Design review of the part shown in the three views and the two pictorial views. Dimensions are in mm from the part's minimum x, y and z. A direction names the side the tool comes from. Coordinates: 2 decimals unless noted, no trailing zeros. Loops run counter-clockwise (first coordinate to the right, second up) from the corner with the lowest first, then second, coordinate; pieces in that order, holes last.
Q1. Wall thickness on probe 1 along Y at (x, z) = (6, 42.5); probe 2 along X at (y, z) = (38, 43.5); probe 3 along Z at (x, y) = (6.5, 13): over which ranges is each line inside the solid? List them lowest first.
Q2. Add section D-D on y = 30. Give the boundary of the cut face in (x, z).
Q3. Add section C-C on z = 47. Give the boundary of the cut face in (x, y).
Q4. Add section A-A on y = 21.25. Give the boundary of the cut face in (x, z).
Q5. For P1, Ø10, axis at x = 22, y = 36.5, coming from the +Z side; P2, Ø3, axis at x = 5.755, y = 5.755, coming from the +Z side, all flat-tipped, find the tip position at first contact; note any pin that passes through.
Q6. Machinability: for the marked faces 1 and 2, which of the approach directions +Z, -Z, +X, -X, +Y, -Y give a long, thin tool a straight path to every point of the face, cutting with its end or side? Answer none if there is none.
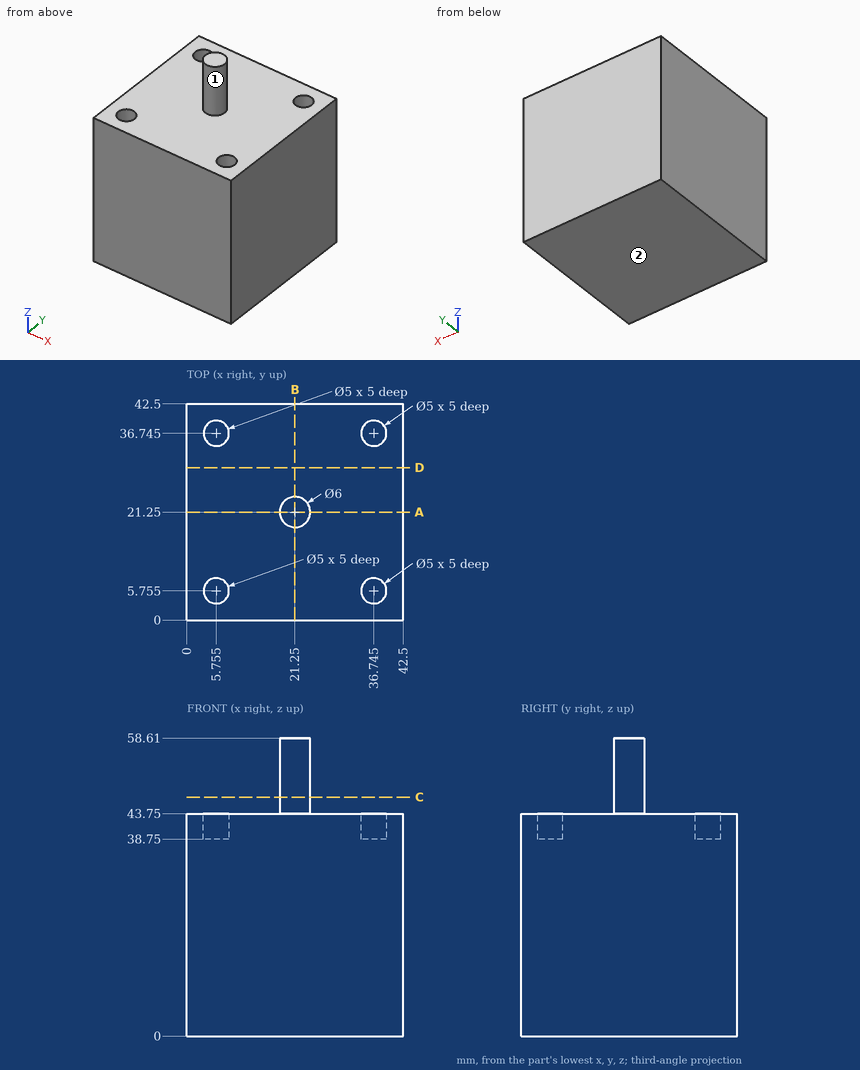
Entries:
1. probe 1: y = 0 to 3.27, 8.24 to 34.26, 39.23 to 42.5
1. probe 2: x = 0 to 3.59, 7.92 to 34.58, 38.91 to 42.5
1. probe 3: z = 0 to 43.75
2. outline: (0, 0) - (42.5, 0) - (42.5, 43.75) - (0, 43.75) - close
3. outline: circle Ø6 at (21.25, 21.25)
4. outline: (0, 0) - (42.5, 0) - (42.5, 43.75) - (24.25, 43.75) - (24.25, 58.61) - (18.25, 58.61) - (18.25, 43.75) - (0, 43.75) - close
5. P1: stops at z = 43.75
5. P2: stops at z = 38.75
6. face 1: +Z
6. face 2: -Z, +X, -X, +Y, -Y
